from build123d import *

# Parameters (mm, degrees)
BOSS_EXTRUDE1_DEPTH = 3
SKETCH2_R           = 7
SKETCH2_R_2         = 6
BOSS_EXTRUDE2_DEPTH = 2


with BuildPart() as part:
    # Sketch1 → Boss-Extrude1 (new body)
    with BuildSketch(Plane(origin=(0, 0, 0), x_dir=(1, 0, 0), z_dir=(0, 1, 0))):
        with BuildLine():
            Line((-38.25, 24.75), (38.25, 24.75))
            ThreePointArc((38.25, 24.75), (40.371320344, 23.871320344), (41.25, 21.75))
            Line((41.25, 21.75), (41.25, -21.75))
            ThreePointArc((41.25, -21.75), (40.371320344, -23.871320344), (38.25, -24.75))
            Line((38.25, -24.75), (-38.25, -24.75))
            ThreePointArc((-38.25, -24.75), (-40.371320344, -23.871320344), (-41.25, -21.75))
            Line((-41.25, -21.75), (-41.25, 21.75))
            ThreePointArc((-41.25, 21.75), (-40.371320344, 23.871320344), (-38.25, 24.75))
        make_face()
    extrude(amount=BOSS_EXTRUDE1_DEPTH)

    # Sketch2 → Boss-Extrude2 (add)
    # profile 1 of 2: a face of its own
    with BuildSketch(Plane(origin=(0, 3, 0), x_dir=(1, 0, 0), z_dir=(0, 1, 0))):
        with Locations(Location((-25, -6.75, 0), (0, 0, 90))):
            Circle(SKETCH2_R)
        with Locations(Location((-25, -6.75, 0), (0, 0, 270))):
            Circle(SKETCH2_R_2, mode=Mode.SUBTRACT)
    # profile 2 of 2: a face of its own
    with BuildSketch(Plane(origin=(0, 3, 0), x_dir=(1, 0, 0), z_dir=(0, 1, 0))):
        with Locations(Location((25, -6.75, 0), (0, 0, 90))):
            Circle(SKETCH2_R)
        with Locations(Location((25, -6.75, 0), (0, 0, 90))):
            Circle(SKETCH2_R_2, mode=Mode.SUBTRACT)
    extrude(amount=BOSS_EXTRUDE2_DEPTH)


solid = part.part
Model file for the job. Use its own axes, mm. A direction names the side the tool comes from. Give positions to 0.01 mm unless a question says otherwise; leave off trailing zeros. Loops run counter-clockwise (first coordinate to the right, second up) from the corner with the lowest first, then second, coordinate; pieces in that order, holes last.
1) Saw through at D-D (z = -3). Write the cut outline in (x, y), plus the area to 4 significant figures.
2) Flat gauge pins, fed straight in: pin 1 Ø13 at (x, z) = (25, 9.5) entering from +Y; pin 2 Ø3 at (x, z) = (8.5, -1.5) entering from +Y. Where does each tip first touch, or does it go through?
3) Tool access for faces 1 (the flat face through (-1, 1, -24.75)), 2 (the cylindrical face through (-24.736, 3.986, 0.756)): list every direction of +Z, -Z, +X, -X, +Y, -Y with a clear straight run to the whole face (end or side of a thin tool).
4) Saw through at B-B (z = 6.75). Write the cut outline in (x, y).
5) Wall check: line 1 (X direction, y = 3.8, z = 6.75); line 2 (Y direction, x = -16, z = 20.5); line 3 (X direction, y = 3.65, z = 4.5). Give the ranges that are in metal, low to high.
6) Saw through at C-C (x = -30). Write the cut outline in (y, z).
7) Pull direction X, two halves, no side cores. Call faces 3 (the cylindrical face through (40.35, 1.48, -23.89)), 4 (the flat face through (31, 5, 5)), 5 (the flat face through (25, 3, 7)): +X half, -X half, draft (parallel to the pull), parting line (faces both ways), or undercut.
8) Saw through at A-A (x = 25). Write the cut outline in (y, z), plus the area to 4 significant figures.
Answer block:
1. outline: (-41.25, 0) - (41.25, 0) - (41.25, 3) - (-41.25, 3) - close
1. area: 247.5 mm2
2. pin 1: stops at y = 5
2. pin 2: stops at y = 3
3. face 1: -Z, +X, -X, +Y, -Y
3. face 2: +Y
4. outline: (-41.25, 0) - (41.25, 0) - (41.25, 3) - (32, 3) - (32, 5) - (31, 5) - (31, 3) - (19, 3) - (19, 5) - (18, 5) - (18, 3) - (-18, 3) - (-18, 5) - (-19, 5) - (-19, 3) - (-31, 3) - (-31, 5) - (-32, 5) - (-32, 3) - (-41.25, 3) - close
5. line 1: x = -32 to -31, -19 to -18, 18 to 19, 31 to 32
5. line 2: y = 0 to 3
5. line 3: x = -31.63 to -30.56, -19.44 to -18.37, 18.37 to 19.44, 30.56 to 31.63
6. outline: (0, -24.75) - (3, -24.75) - (3, 1.85) - (5, 1.85) - (5, 3.43) - (3, 3.43) - (3, 10.07) - (5, 10.07) - (5, 11.65) - (3, 11.65) - (3, 24.75) - (0, 24.75) - close
7. face 3: +X half
7. face 4: draft
7. face 5: undercut
8. outline: (0, -24.75) - (3, -24.75) - (3, -0.25) - (5, -0.25) - (5, 0.75) - (3, 0.75) - (3, 12.75) - (5, 12.75) - (5, 13.75) - (3, 13.75) - (3, 24.75) - (0, 24.75) - close
8. area: 152.5 mm2
